Geometry: final body of the model. Coordinates: model frame, mm. A direction names the side the tool comes from. Give positions to 0.01 mm unless a question says otherwise; leave off trailing zeros. Write each loop counter-clockwise with the first axis right and the second up, starting at its lowest first coordinate (ties: lowest second). Pieces come first, ordered by that corner, then holes. Notation, with made-up numbers: M 21.5,49.5 L 60.5,49.5 A19 ccw 60.5,77.5 Z; hole C -22,36.5 d8. An arc over 180 degrees is marked long. Use a Markdown table: item, result. Add a question column.
1) Section B-B on x = 33. Return the cut outline in (y, z), then the cut area to 3 significant figures.
2) Set-up query: faces 1 (the flat face through (112, 126.057, -2)), 2 (the cylindrical face through (116.135, 51.498, -4.437)), 3 (the flat face through (50.87, 137.44, -9)). Return all of +Z, -Z, +X, -X, +Y, -Y with unobstructed straight access to the full face (end or side cutting, diameter ignored); none if empty.
3) Section C-C on y = 66.5. Return the cut outline in (x, z).
4) Line query: line 1 (Y direction, x = 13, z = 1.1) (3 decimals); line 2 (Y direction, x = 198.31, z = -3.5); line 3 (Y direction, x = 197, z = -4). Output: solid intervals per line, ascending.
5) Pin query (flat end, axial travel): pin 1 (2.5 mm diameter, centred on x = 25.79, y = 118.58, fed in from -Z); pin 2 (7 mm diameter, centred on x = 156.21, y = 53.6, fed in from +Z); pin 3 (1.5 mm diameter, centred on y = 136, z = -3.5, fed in from -X); pin 4 (2.5 mm diameter, centred on y = 127.5, z = -3, fed in from +X). Return the tip coordinate at first contact, or that it passes through.
6) Draft query along Y for faces 4 (the cylindrical face through (181.015, 124.104, 1.479)), 5 (the flat face through (198.3, 54.5, -9)). Return one class per face: +Y half, -Y half, draft (parallel to the pull), parting line (faces both ways), or undercut.
7) Section A-A on y = 29.5. Return the cut outline in (x, z), then the cut area to 3 significant figures.
Autodesk Fusion 360 part; units mm, degrees
sketch "Sketch1" plane through (0, 0, 0) normal (0, 0, 1) x (1, 0, 0)
  line L0 (0, 0) -> (225, 0)
  line L1 (225, 0) -> (225, 158.6)
  line L2 (225, 158.6) -> (0, 158.6)
  line L3 (0, 158.6) -> (0, 0)
  dimension "d1" = 158.6
  dimension "d2" = 225
extrude "Extrude1" add sketch "Sketch1" along normal blind 3
sketch "Sketch2" plane through (0, 0, 3) normal (0, 0, 1) x (-1, 0, 0)
  line L0 (0, -158.6) -> (0, 0)
  line L1 (0, 0) -> (-225, 0)
  line L2 (-225, 0) -> (-225, -158.6)
  line L3 (-225, -158.6) -> (0, -158.6)
  circle A0 centre (-13, -123.6) radius 3.25
  dimension "d5" = 13
  dimension "d6" = 35
  dimension "d7" = 6.5
hole "Hole1" at (13, 123.6, 3) direction (0, 0, -1) diameter 7.75 end through all
pattern_linear "R-Pattern4" count 4 spacing 23.3333 along (0, -1, 0) count 8 spacing 28.6429 along (1, 0, 0) of "Hole1"
sketch "MountingPostsSketch" plane through (0, 0, 0) normal (0, 0, 1) x (1, 0, 0)
  circle A0 centre (25.79, 118.58) radius 4
  circle A1 centre (25.79, 50.49) radius 4
  circle A2 centre (51.81, 136.5) radius 4
  circle A3 centre (112.44, 99.27) radius 4
  circle A4 centre (112.44, 53.03) radius 4
  circle A5 centre (138.38, 144.98) radius 4
  circle A6 centre (198.31, 117.8) radius 4
  circle A7 centre (198.31, 56.27) radius 4
  dimension "d47" = 8
  dimension "d48" = 8
  dimension "d50" = 8
  dimension "d51" = 8
  dimension "d52" = 8
  dimension "d53" = 8
  dimension "d54" = 8
  dimension "d55" = 8
extrude "Extrude2" add sketch "MountingPostsSketch" against normal blind 9
sketch "M3HolesSketch" plane through (0, 0, 0) normal (0, 0, 1) x (1, 0, 0)
  circle A0 centre (25.79, 118.58) radius 1.6
  circle A1 centre (25.79, 50.49) radius 1.6
  circle A2 centre (51.91, 136) radius 1.6
  circle A3 centre (112.54, 99.27) radius 1.6
  circle A4 centre (112.44, 53.03) radius 1.6
  circle A5 centre (138.38, 144.98) radius 1.6
  circle A6 centre (198.31, 117.8) radius 1.6
  circle A7 centre (198.31, 56.27) radius 1.6
  circle A8 centre (198.31, 117.8) radius 4
  dimension "d49" = 8
ref_plane "WorkPlane1" through (0, 0, 2) normal (0, 0, 1) x (1, 0, 0)
sketch "OLED_Opening_Sketch" plane through (0, 0, 2) normal (0, 0, 1) x (1, 0, 0)
  line L0 (99.5, 135.6) -> (125.5, 135.6)
  line L1 (125.5, 135.6) -> (125.5, 150.35)
  line L2 (125.5, 150.35) -> (99.5, 150.35)
  line L3 (99.5, 150.35) -> (99.5, 135.6)
extrude "Extrude4" cut sketch "OLED_Opening_Sketch" along normal through all and the other way through all
ref_plane "WorkPlane2" through (0, 0, 2) normal (0, 0, 1) x (1, 0, 0)
sketch "MountingHoles_Sketch" plane through (0, 0, 2) normal (0, 0, 1) x (1, 0, 0)
  circle A0 centre (100.5, 153.1) radius 1.3
  circle A1 centre (124.5, 153.1) radius 1.3
  dimension "d56" = 2.6
  dimension "d57" = 2.6
extrude "Extrude5" cut sketch "MountingHoles_Sketch" along normal blind 15 and the other way blind 3
sketch "Sketch7" plane through (0, 0, 0) normal (0, 0, -1) x (1, 0, 0)
  line L0 (125.5, -150.35) -> (99.5, -150.35)
  line L1 (99.5, -150.35) -> (99.5, -135.6)
  line L2 (99.5, -135.6) -> (125.5, -135.6)
  line L3 (125.5, -135.6) -> (125.5, -150.35)
  circle A0 centre (213.5003, -76.9334) radius 3.875
  circle A1 centre (213.5003, -123.6) radius 3.875
  circle A2 centre (184.8574, -76.9334) radius 3.875
  circle A3 centre (184.8574, -123.6) radius 3.875
  circle A4 centre (156.2145, -76.9334) radius 3.875
  circle A5 centre (156.2145, -123.6) radius 3.875
  circle A6 centre (127.5716, -76.9334) radius 3.875
  circle A7 centre (127.5716, -123.6) radius 3.875
  circle A8 centre (98.9287, -76.9334) radius 3.875
  circle A9 centre (98.9287, -123.6) radius 3.875
  circle A10 centre (70.2858, -76.9334) radius 3.875
  circle A11 centre (70.2858, -123.6) radius 3.875
  line L4 (0, 0) -> (0, -158.6)
  line L5 (0, -158.6) -> (225, -158.6)
  line L6 (225, -158.6) -> (225, 0)
  line L7 (225, 0) -> (0, 0)
  circle A12 centre (13, -123.6) radius 3.875
  circle A13 centre (13, -100.2667) radius 3.875
  circle A14 centre (13, -76.9334) radius 3.875
  circle A15 centre (13, -53.6001) radius 3.875
  circle A16 centre (41.6429, -123.6) radius 3.875
  circle A17 centre (41.6429, -100.2667) radius 3.875
  circle A18 centre (41.6429, -76.9334) radius 3.875
  circle A19 centre (41.6429, -53.6001) radius 3.875
  circle A20 centre (70.2858, -100.2667) radius 3.875
  circle A21 centre (70.2858, -53.6001) radius 3.875
  circle A22 centre (98.9287, -100.2667) radius 3.875
  circle A23 centre (98.9287, -53.6001) radius 3.875
  circle A24 centre (127.5716, -100.2667) radius 3.875
  circle A25 centre (127.5716, -53.6001) radius 3.875
  circle A26 centre (156.2145, -100.2667) radius 3.875
  circle A27 centre (156.2145, -53.6001) radius 3.875
  circle A28 centre (184.8574, -100.2667) radius 3.875
  circle A29 centre (184.8574, -53.6001) radius 3.875
  circle A30 centre (213.5003, -100.2667) radius 3.875
  circle A31 centre (213.5003, -53.6001) radius 3.875
  line L8 (118.5096, -127.6004) -> (106.547, -127.6004)
  line L9 (106.547, -127.6004) -> (106.547, -126.0574)
  line L10 (106.547, -126.0574) -> (118.5096, -126.0574)
  line L11 (118.5096, -126.0574) -> (118.5096, -127.6004)
  circle A32 centre (138.38, -144.98) radius 4
  circle A33 centre (51.81, -136.5) radius 4
  circle A34 centre (112.44, -99.27) radius 4
  circle A35 centre (198.31, -117.8) radius 4
  circle A36 centre (112.44, -53.03) radius 4
  circle A37 centre (25.79, -50.49) radius 4
  circle A38 centre (25.79, -118.58) radius 4
  circle A39 centre (198.31, -56.27) radius 4
  circle A40 centre (124.5, -153.1) radius 1.3
  circle A41 centre (100.5, -153.1) radius 1.3
extrude "Extrude6" add sketch "Sketch7" along normal blind 3 contours L8 L9 L10 L11
sketch "Sketch8" plane through (0, 0, -3) normal (0, 0, -1) x (1, 0, 0)
  line L0 (118.5096, -126.0574) -> (106.547, -126.0574)
  line L1 (106.547, -126.0574) -> (106.547, -127.6004)
  line L2 (106.547, -127.6004) -> (118.5096, -127.6004)
  line L3 (118.5096, -127.6004) -> (118.5096, -126.0574)
  line L4 (118.5096, -126.0574) -> (106.4856, -126.0574)
  line L5 (106.4856, -126.0574) -> (106.4856, -129.1746)
  line L6 (106.4856, -129.1746) -> (118.5096, -129.1746)
  line L7 (118.5096, -129.1746) -> (118.5096, -126.0574)
extrude "Extrude3" cut sketch "M3HolesSketch" against normal blind 9 contours A0 | A1 | A2 | A3 | A4 | A5 | A6 | A7
extrude "Extrude7" add sketch "Sketch8" along normal blind 1.5
chamfer "Chamfer1" distance 1 angle 45 4 edges at (225, 79.3, 3) (112.5, 158.6, 3) (0, 79.3, 3) (112.5, 0, 3)
chamfer "Chamfer2" distance 1 angle 45 4 edges at (112.5, 135.6, 3) (99.5, 142.975, 3) (112.5, 150.35, 3) (125.5, 142.975, 3)
sketch "Sketch9" plane through (0, 0, 3) normal (0, 0, 1) x (-1, 0, 0)
  line L0 (-1, -157.6) -> (-1, -1)
  line L1 (-1, -1) -> (-224, -1)
  line L2 (-224, -1) -> (-224, -157.6)
  line L3 (-224, -157.6) -> (-1, -157.6)
  circle A0 centre (-213.5003, -76.9334) radius 3.875
  circle A1 centre (-213.5003, -123.6) radius 3.875
  circle A2 centre (-184.8574, -76.9334) radius 3.875
  circle A3 centre (-184.8574, -123.6) radius 3.875
  circle A4 centre (-156.2145, -76.9334) radius 3.875
  circle A5 centre (-156.2145, -123.6) radius 3.875
  circle A6 centre (-127.5716, -76.9334) radius 3.875
  circle A7 centre (-127.5716, -123.6) radius 3.875
  circle A8 centre (-98.9287, -76.9334) radius 3.875
  circle A9 centre (-98.9287, -123.6) radius 3.875
  circle A10 centre (-70.2858, -76.9334) radius 3.875
  circle A11 centre (-70.2858, -123.6) radius 3.875
  circle A12 centre (-13, -123.6) radius 3.875
  circle A13 centre (-13, -100.2667) radius 3.875
  circle A14 centre (-13, -76.9334) radius 3.875
  circle A15 centre (-13, -53.6001) radius 3.875
  circle A16 centre (-41.6429, -123.6) radius 3.875
  circle A17 centre (-41.6429, -100.2667) radius 3.875
  circle A18 centre (-41.6429, -76.9334) radius 3.875
  circle A19 centre (-41.6429, -53.6001) radius 3.875
  circle A20 centre (-70.2858, -100.2667) radius 3.875
  circle A21 centre (-70.2858, -53.6001) radius 3.875
  circle A22 centre (-98.9287, -100.2667) radius 3.875
  circle A23 centre (-98.9287, -53.6001) radius 3.875
  circle A24 centre (-127.5716, -100.2667) radius 3.875
  circle A25 centre (-127.5716, -53.6001) radius 3.875
  circle A26 centre (-156.2145, -100.2667) radius 3.875
  circle A27 centre (-156.2145, -53.6001) radius 3.875
  circle A28 centre (-184.8574, -100.2667) radius 3.875
  circle A29 centre (-184.8574, -53.6001) radius 3.875
  circle A30 centre (-213.5003, -100.2667) radius 3.875
  circle A31 centre (-213.5003, -53.6001) radius 3.875
  circle A32 centre (-124.5, -153.1) radius 1.3
  circle A33 centre (-100.5, -153.1) radius 1.3
  line L4 (-126.5, -134.6) -> (-98.5, -134.6)
  line L5 (-98.5, -134.6) -> (-98.5, -151.35)
  line L6 (-98.5, -151.35) -> (-126.5, -151.35)
  line L7 (-126.5, -151.35) -> (-126.5, -134.6)
  circle A34 centre (-213.6, -30) radius 4
  circle A35 centre (-12.6309, -29.642) radius 4
  dimension "d58" = 8
  dimension "d62" = 8
hole "Hole2" at (213.6, 30, 3) direction (0, 0, -1) diameter 8 depth 3 tip angle 118
hole "Hole3" at (12.6309, 29.642, 3) direction (0, 0, -1) diameter 7 depth 3 tip angle 118
equation "d22 = -( 9 mm )"
equation "d24 = -( 9 mm )"
Found:
| question | item | result |
|---|---|---|
| 1 | outline | M 0,0 L 158.6,0 L 158.6,2 L 157.6,3 L 1,3 L 0,2 Z |
| 1 | area | 475 mm² |
| 2 | face 1 | -Z, +X, -X |
| 2 | face 2 | -Z |
| 2 | face 3 | -Z, +X, -X, +Y, -Y |
| 3 | outline | M 0,0 L 225,0 L 225,2 L 224,3 L 1,3 L 0,2 Z |
| 4 | line 1 | 0 to 26.162, 33.122 to 49.725, 57.475 to 73.058, 80.808 to 96.392, 104.142 to 119.725, 127.475 to 158.6 |
| 4 | line 2 | 52.27 to 54.67, 57.87 to 60.27, 113.8 to 116.2, 119.4 to 121.8 |
| 4 | line 3 | 52.49 to 55.35, 57.19 to 60.05, 114.02 to 116.88, 118.72 to 121.58 |
| 5 | pin 1 | z = 0 |
| 5 | pin 2 | through |
| 5 | pin 3 | x = 47.81 |
| 5 | pin 4 | x = 118.51 |
| 6 | face 4 | undercut |
| 6 | face 5 | draft |
| 7 | outline | M 0,0 L 9.13,0 L 9.13,3 L 1,3 L 0,2 Z; M 16.13,0 L 209.63,0 L 209.63,3 L 16.13,3 Z; M 217.57,0 L 225,0 L 225,2 L 224,3 L 217.57,3 Z |
| 7 | area | 629 mm² |
